from build123d import *

# Parameters (mm, degrees)
F0_R     = 4
F1_DEPTH = 100
F2_SIZE  = 0.5
F3_SIZE  = 0.5


with BuildPart() as f1:
    # F0 (on Front) → F1 (new body)
    with BuildSketch(Plane.XZ):
        Circle(F0_R)
    extrude(amount=F1_DEPTH)

    # F2
    f2_edges = [f1.edges().sort_by_distance(p)[0] for p in [
        (-4, 0, 0),
    ]]
    chamfer(f2_edges, length=F2_SIZE)

    # F3
    f3_edges = [f1.edges().sort_by_distance(p)[0] for p in [
        (-4, -100, 0),
    ]]
    chamfer(f3_edges, length=F3_SIZE)


solid = f1.part
Part model, mm, in its own coordinate system. Give positions to 0.01 mm unless a question says otherwise; leave off trailing zeros. Loops run counter-clockwise (first coordinate to the right, second up) from the corner with the lowest first, then second, coordinate; pieces in that order, holes last. Notation, with made-up numbers: (26.5, -39) -> (50.5, -39) arc R8 cw to (50.5, -28) -> close; hole circle Ø1 at (80, -12.75). An arc over 180 degrees is marked (long way). Write each question's results on one line, items separated by ' | '. Start each with the question number.
Q1. Wall check: L1, parallel to X at y = -55.5, z = -0.25; L2, parallel to X at y = -45.5, z = 1. Give the ranges that are in metal, low to high.
Q2. Pin check, flat tip, straight feed: P1, Ø4, axis at y = -79, z = 2.5, coming from the +X side. Stop position of the tip, or through.
Q3. Band-saw the part on A-A on y = -75.5. List the corners of the cut face in (x, z), plus the area to 3 significant figures.
Results are:
1) L1: x = -3.99 to 3.99 | L2: x = -3.87 to 3.87
2) P1: stops at x = 3.97
3) outline: circle Ø8 at (0, 0) | area: 50.3 mm²
